Source: CAD feature listing. Evaluate the final solid. Frame: model axes, mm. A direction names the side the tool comes from. Give positions to 0.01 mm unless a question says otherwise; leave off trailing zeros. Loops run counter-clockwise (first coordinate to the right, second up) from the corner with the lowest first, then second, coordinate; pieces in that order, holes last. Notation, with made-up numbers: M 63,55 L 114,55 A19 ccw 114,66 Z; hole C -13,48 d10. An arc over 180 degrees is marked long. Write item = value, one per line.
from build123d import *

# Parameters (mm, degrees)
F0_W     = 172
F0_H     = 306
F1_DEPTH = 2
F0_H_2   = 2
F2_DEPTH = 62
F3_DEPTH = 62


with BuildPart() as f1:
    # F0 (on Front) → F1 (new body)
    with BuildSketch(Plane.XZ):
        Rectangle(F0_W, F0_H)
    extrude(amount=F1_DEPTH)

    # F0 (on Front) → F2 (join)
    with BuildSketch(Plane.XZ):
        with Locations((0, 154)):
            Rectangle(F0_W, F0_H_2)
    extrude(amount=F2_DEPTH)

    # F0 (on Front) → F3 (join)
    with BuildSketch(Plane.XZ):
        with Locations((0, -154)):
            Rectangle(F0_W, F0_H_2)
    extrude(amount=F3_DEPTH)


solid = f1.part
1. First-contact query: pin 1 Ø2 at (x, z) = (-57.5, -3.5) entering from -Y. Flat tip, straight axial feed; report the tip coordinate or a pass-through.
Derived:
pin_1 = -2
2. Cut plane A-A, the plane y = -43.5. Return the cut outline in (x, z).
Derived:
outline = M -86,-155 L 86,-155 L 86,-153 L -86,-153 Z; M -86,153 L 86,153 L 86,155 L -86,155 Z
3. Reachability of faces 5 (the flat face through (-1, -2, 2)), 6 (the flat face through (-86, -1, -1)) from +Z, -Z, +X, -X, +Y, -Y: full face, straight path, thin tool, end or side. Return the list, or none.
Derived:
face_5 = +X, -X, -Y
face_6 = +Z, -Z, -X, +Y, -Y
4. Cut plane B-B, the plane x = -48.5. Return the cut outline in (y, z), then the cut area to 3 significant figures.
Derived:
outline = M -62,-155 L 0,-155 L 0,155 L -62,155 L -62,153 L -2,153 L -2,-153 L -62,-153 Z
area = 860 mm²
5. Cut plane C-C, the plane z = -116. Return the cut outline in (x, y), then the cut area to 3 significant figures.
Derived:
outline = M -86,-2 L 86,-2 L 86,0 L -86,0 Z
area = 344 mm²
6. Pull-direction query (Z, two-part tool) for faces 1 (the flat face through (-1, 0, 2)), 2 (the flat face through (-1, -31, 155)), 3 (the flat face through (-1, -32, -153)), 4 (the flat face through (-1, -32, 153)); classes: +Z half, -Z half, draft (parallel to the pull), parting line (faces both ways), or undercut.
Derived:
face_1 = draft
face_2 = +Z half
face_3 = undercut
face_4 = undercut
7. Material intervals for probe 1 along Z at (x, y) = (5.5, -49.5); probe 2 along Y at (x, z) = (-61, 138), sorted ascending. Write a range as from..to.
Derived:
probe_1 = -155..-153, 153..155
probe_2 = -2..0
